The listing builds one solid part. Answer for the finished solid, in the listing's coordinates (mm). Face numbers are marked on the shaded views. A direction names the side the tool comes from. Round coordinates to 2 decimals unless told otherwise and drop trailing zeros. Loops run counter-clockwise (first coordinate to the right, second up) from the corner with the lowest first, then second, coordinate; pieces in that order, holes last. Notation, with made-up numbers: (-26.5, -21) -> (-11.5, -21) arc R18 cw to (-11.5, -11) -> close; hole circle Ø2 at (17.25, -26.75). An arc over 180 degrees is marked (long way). One line per question, with ' | ' between items.
from build123d import *

# Parameters (mm, degrees)
SKETCH1_R           = 1.65
BOSS_EXTRUDE1_DEPTH = 32
CUT_EXTRUDE3_START  = -22
CUT_EXTRUDE3_DEPTH  = 22
CUT_EXTRUDE1_DEPTH  = 26
SKETCH3_W           = 76.8
SKETCH3_H           = 51.4
CUT_EXTRUDE2_DEPTH  = 23.6
CUT_EXTRUDE4_REACH  = 76.888
SKETCH5_R           = 1.65
CUT_EXTRUDE5_DEPTH  = 4


with BuildPart() as part:
    # Sketch1 → Boss-Extrude1 (new body)
    with BuildSketch(Plane.XY):
        with BuildLine():
            Line((-40.01, -32.7), (-40.01, 25.7))
            ThreePointArc((-40.01, 25.7), (-39.538441918, 26.838441918), (-38.4, 27.31))
            Line((-38.4, 27.31), (38.4, 27.31))
            ThreePointArc((38.4, 27.31), (39.538441918, 26.838441918), (40.01, 25.7))
            Line((40.01, 25.7), (40.01, -32.7))
            ThreePointArc((40.01, -32.7), (39.538441918, -33.838441918), (38.4, -34.31))
            Line((38.4, -34.31), (-38.4, -34.31))
            ThreePointArc((-38.4, -34.31), (-39.538441918, -33.838441918), (-40.01, -32.7))
        make_face()
        with Locations((-34.925, 22.225)):
            Circle(SKETCH1_R, mode=Mode.SUBTRACT)
        with Locations((-34.925, -22.225)):
            Circle(SKETCH1_R, mode=Mode.SUBTRACT)
        with Locations((34.925, 22.225)):
            Circle(SKETCH1_R, mode=Mode.SUBTRACT)
        with Locations((34.925, -22.225)):
            Circle(SKETCH1_R, mode=Mode.SUBTRACT)
    extrude(amount=BOSS_EXTRUDE1_DEPTH)

    # Sketch4 → Cut-Extrude3 (cut)
    with BuildSketch(Plane.XY.offset(32).offset(CUT_EXTRUDE3_START)):
        with BuildLine():
            Line((-38.4, -27.31), (38.4, -27.31))
            ThreePointArc((38.4, -27.31), (39.538441918, -27.781558082), (40.01, -28.92))
            Line((40.01, -28.92), (40.01, 25.7))
            ThreePointArc((40.01, 25.7), (39.538441918, 26.838441918), (38.4, 27.31))
            Line((38.4, 27.31), (-38.4, 27.31))
            ThreePointArc((-38.4, 27.31), (-39.538441918, 26.838441918), (-40.01, 25.7))
            Line((-40.01, 25.7), (-40.01, -28.92))
            ThreePointArc((-40.01, -28.92), (-39.538441918, -27.781558082), (-38.4, -27.31))
        make_face()
    extrude(amount=CUT_EXTRUDE3_DEPTH, mode=Mode.SUBTRACT)

    # Sketch2 → Cut-Extrude1 (cut)
    with BuildSketch(Plane.XY.offset(32)):
        with BuildLine():
            Line((-31.665, 25.7), (31.665, 25.7))
            Line((31.665, 25.7), (31.665, 22.225))
            ThreePointArc((31.665, 22.225), (32.619831893, 19.919831893), (34.925, 18.965))
            Line((34.925, 18.965), (38.4, 18.965))
            Line((38.4, 18.965), (38.4, -18.965))
            Line((38.4, -18.965), (34.925, -18.965))
            ThreePointArc((34.925, -18.965), (32.619831893, -19.919831893), (31.665, -22.225))
            Line((31.665, -22.225), (31.665, -25.7))
            Line((31.665, -25.7), (-31.665, -25.7))
            Line((-31.665, -25.7), (-31.665, -22.225))
            ThreePointArc((-31.665, -22.225), (-32.619831893, -19.919831893), (-34.925, -18.965))
            Line((-34.925, -18.965), (-38.4, -18.965))
            Line((-38.4, -18.965), (-38.4, 18.965))
            Line((-38.4, 18.965), (-34.925, 18.965))
            ThreePointArc((-34.925, 18.965), (-32.619831893, 19.919831893), (-31.665, 22.225))
            Line((-31.665, 22.225), (-31.665, 25.7))
        make_face()
    extrude(amount=-CUT_EXTRUDE1_DEPTH, mode=Mode.SUBTRACT)

    # Sketch3 → Cut-Extrude2 (cut)
    with BuildSketch(Plane.XY.offset(32)):
        Rectangle(SKETCH3_W, SKETCH3_H)
    extrude(amount=-CUT_EXTRUDE2_DEPTH, mode=Mode.SUBTRACT)

    # Sketch5 → Cut-Extrude4 (cut, up to next)
    with BuildSketch(Plane(origin=(0, -27.31, 0), x_dir=(1, 0, 0), z_dir=(0, 1, 0)), mode=Mode.PRIVATE) as cut_extrude4_sk1:
        with Locations(Location((-35.51, -16, 0), (0, 0, 180))):
            Circle(SKETCH5_R)
    cut_extrude4_tool1 = extrude(cut_extrude4_sk1.sketch, amount=-CUT_EXTRUDE4_REACH, mode=Mode.PRIVATE) & part.part
    # Sketch5 → Cut-Extrude4 (cut, up to next)
    with BuildSketch(Plane(origin=(0, -27.31, 0), x_dir=(1, 0, 0), z_dir=(0, 1, 0)), mode=Mode.PRIVATE) as cut_extrude4_sk2:
        with Locations(Location((35.51, -16, 0), (0, 0, 180))):
            Circle(SKETCH5_R)
    cut_extrude4_tool2 = extrude(cut_extrude4_sk2.sketch, amount=-CUT_EXTRUDE4_REACH, mode=Mode.PRIVATE) & part.part
    add(cut_extrude4_tool1.solids().sort_by_distance((-35.51, -27.31, 16))[0], mode=Mode.SUBTRACT)
    add(cut_extrude4_tool2.solids().sort_by_distance((35.51, -27.31, 16))[0], mode=Mode.SUBTRACT)

    # Sketch6 → Cut-Extrude5 (cut)
    with BuildSketch(Plane(origin=(0, -27.31, 0), x_dir=(1, 0, 0), z_dir=(0, 1, 0))):
        Polygon((-35.51, -19.348631561), (-32.61, -17.674315781), (-32.61, -14.325684219), (-35.51, -12.651368439), (-38.41, -14.325684219), (-38.41, -17.674315781), align=None)
        Polygon((35.51, -19.348631561), (38.41, -17.674315781), (38.41, -14.325684219), (35.51, -12.651368439), (32.61, -14.325684219), (32.61, -17.674315781), align=None)
    extrude(amount=-CUT_EXTRUDE5_DEPTH, mode=Mode.SUBTRACT)


solid = part.part
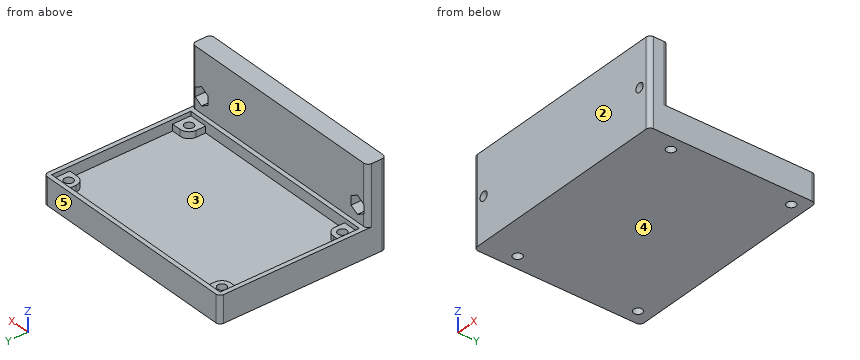
Q1. A cutting plane is placed at B-B on x = 29. Give the vertices of the cut face in (y, z), plus the area to 3 significant figures.
Numbers:
outline: (-34.31, 0) -> (27.31, 0) -> (27.31, 10) -> (25.7, 10) -> (25.7, 6) -> (-25.7, 6) -> (-25.7, 10) -> (-27.31, 10) -> (-27.31, 32) -> (-34.31, 32) -> close | area: 565 mm^2
Q2. A cutting plane is placed at A-A on z = 16. Give the vertices of the cut face in (x, y), plus the area to 3 significant figures.
Numbers:
outline: (-40.01, -32.7) arc R1.61 ccw to (-38.4, -34.31) -> (-37.16, -34.31) -> (-37.16, -31.31) -> (-38.41, -31.31) -> (-38.41, -27.31) arc R1.61 ccw to (-40.01, -28.92) -> close; (-33.86, -34.31) -> (33.86, -34.31) -> (33.86, -31.31) -> (32.61, -31.31) -> (32.61, -27.31) -> (-32.61, -27.31) -> (-32.61, -31.31) -> (-33.86, -31.31) -> close; (37.16, -34.31) -> (38.4, -34.31) arc R1.61 ccw to (40.01, -32.7) -> (40.01, -28.92) arc R1.61 ccw to (38.41, -27.31) -> (38.41, -31.31) -> (37.16, -31.31) -> close | area: 492 mm^2
Q3. For a pull along Y with two mould halves and no side action, classify the marked faces 3, 4 and 5 as pulls with the +Y half, pulls with the -Y half, needs draft (parallel to the pull), parting line crosses it, or undercut.
Numbers:
face 3: undercut | face 4: needs draft | face 5: pulls with the +Y half
Q4. Given pin 1 Ø6.5 at (x, z) = (16.5, 20) entering from +Y; pin 2 Ø1.7 at (x, z) = (35.5, 17) entering from +Y; pin 3 Ø5.5 at (x, y) = (-34.5, -21.5) entering from +Z, each flat-ended and moving along its own axis, determine where each tip first touches the part or whether it passes through.
Numbers:
pin 1: y = -27.31 | pin 2: y = -31.31 | pin 3: z = 8.4
Q5. For the marked faces 1 and 2, determine the directions among +Z, -Z, +X, -X, +Y, -Y from which every point of the face is accessible in a straight line to the end or side of a thin tool.
Numbers:
face 1: +Z, +X, -X, +Y | face 2: +Z, -Z, +X, -X, -Y
Q6. A cutting plane is placed at C-C on y = -18. Give the vertices of the cut face in (x, z), plus the area to 3 significant figures.
Numbers:
outline: (-40.01, 0) -> (40.01, 0) -> (40.01, 10) -> (38.4, 10) -> (38.4, 6) -> (-38.4, 6) -> (-38.4, 10) -> (-40.01, 10) -> close | area: 493 mm^2
Q7. Find the intervals of material crossed by line 1 (Z direction, x = 35.51, y = -32.9); line 2 (Y direction, x = 1, z = 8); line 3 (Z direction, x = 23.5, y = 10.5), in increasing order. Write a range as from..to.
Numbers:
line 1: 0..14.35, 17.65..32 | line 2: -34.31..-25.7, 25.7..27.31 | line 3: 0..6
